Verification items for this drawing (mm, ordinates from the low corner). Coordinates: 2 decimals unless noted, no trailing zeros. Write each loop counter-clockwise with the first axis right and the second up, starting at its lowest first coordinate (ties: lowest second). Pieces come first, ordered by that corner, then holes.
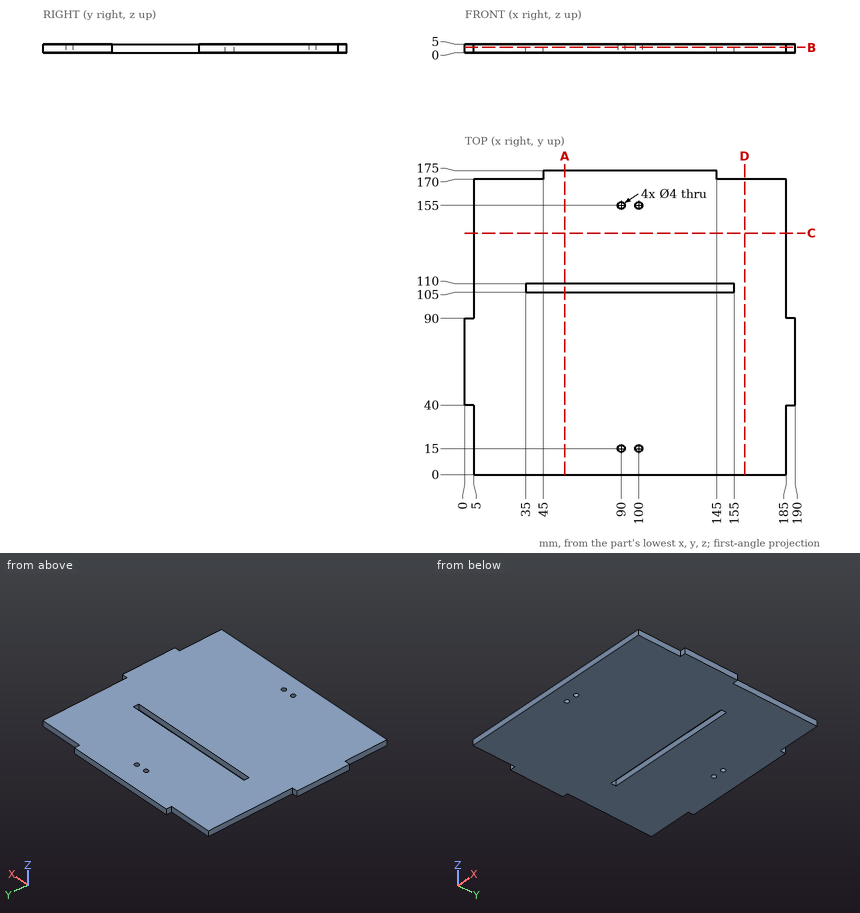
1. Sectioned sample at A-A, the plane x = 57.5. Record the boundary of the cut face in (y, z), and give its area (3 significant figures).
Computed values:
outline: (0, 0) - (105, 0) - (105, 5) - (0, 5) - close; (110, 0) - (175, 0) - (175, 5) - (110, 5) - close
area: 850 mm2
2. Sectioned sample at C-C, the plane y = 139. Record the boundary of the cut face in (x, z).
Computed values:
outline: (5, 0) - (185, 0) - (185, 5) - (5, 5) - close
3. Gauge pin test, flat ends, axial feed: pin 1 Ø2.5 at (y, z) = (107.5, 1.5) entering from -X; pin 2 Ø1.5 at (y, z) = (173.5, 3) entering from +X; pin 3 Ø1.5 at (y, z) = (148, 2) entering from +X; pin 4 Ø3 at (x, y) = (90, 155) entering from -Z. Record the tip position at first contact, or that the pin passes through.
Computed values:
pin 1: stops at x = 5
pin 2: stops at x = 145
pin 3: stops at x = 185
pin 4: passes through
4. Thickness scan on line 1 along Y through (x, z) = (100, 2.8); line 2 along X through (y, z) = (155, 1.7); line 3 along Y through (x, z) = (54.5, 4.4). Record the ranges inside material, lowest first.
Computed values:
line 1: y = 0 to 13, 17 to 105, 110 to 153, 157 to 175
line 2: x = 5 to 88, 92 to 98, 102 to 185
line 3: y = 0 to 105, 110 to 175
5. Sectioned sample at B-B, the plane z = 3.1. Record the boundary of the cut face in (x, y), and give its area (3 significant figures).
Computed values:
outline: (0, 40) - (5, 40) - (5, 0) - (185, 0) - (185, 40) - (190, 40) - (190, 90) - (185, 90) - (185, 170) - (145, 170) - (145, 175) - (45, 175) - (45, 170) - (5, 170) - (5, 90) - (0, 90) - close; hole (35, 105) - (155, 105) - (155, 110) - (35, 110) - close; hole circle Ø4 at (90, 15); hole circle Ø4 at (90, 155); hole circle Ø4 at (100, 15); hole circle Ø4 at (100, 155)
area: 30,900 mm2
6. Sectioned sample at D-D, the plane x = 161. Record the boundary of the cut face in (y, z), and give its area (3 significant figures).
Computed values:
outline: (0, 0) - (170, 0) - (170, 5) - (0, 5) - close
area: 850 mm2
